from build123d import *

# Parameters (mm, degrees)
SKETCH1_R               = 7.5
BOSS_EXTRUDE1_DEPTH     = 56
SKETCH2_W               = 10
SKETCH2_H               = 16
CUT_EXTRUDE1_DEPTH      = 10
CUT_EXTRUDE4_DEPTH      = 57.995613866
CUT_EXTRUDE4_DEPTH_BACK = 57.995613866
CUT_EXTRUDE5_DEPTH      = 57.995613991
CUT_EXTRUDE5_DEPTH_BACK = 57.995613991
SKETCH4_R               = 1.5
FILLET1_R               = 0.1
SKETCH5_W               = 7.5
SKETCH5_H               = 20
SKETCH6_W               = 40
SKETCH6_H               = 40
BOSS_EXTRUDE2_DEPTH     = 5


with BuildPart() as part:
    # Sketch1 → Boss-Extrude1 (new body)
    with BuildSketch(Plane.XY):
        Circle(SKETCH1_R)
    extrude(amount=BOSS_EXTRUDE1_DEPTH)

    # Sketch2 → Cut-Extrude1 (cut)
    with BuildSketch(Plane.XY.offset(56)):
        Rectangle(SKETCH2_W, SKETCH2_H)
    extrude(amount=-CUT_EXTRUDE1_DEPTH, mode=Mode.SUBTRACT)

    # Sketch3 → Cut-Extrude4 (cut, two sides: drawn at the far end of the back side and taken through both)
    with BuildSketch(Plane(origin=(0, 0, 0), x_dir=(0, 0, -1), z_dir=(1, 0, 0)).offset(-CUT_EXTRUDE4_DEPTH_BACK)):
        with BuildLine():
            Line((-46, -114.267763227), (-46, -7.5))
            Line((-46, -7.5), (-46, -5.590169944))
            Line((-46, -5.590169944), (-52.952744721, -3.885047998))
            ThreePointArc((-52.952744721, -3.885047998), (-55.999999999, -0.000262165), (-52.952923855, 3.884664175))
            Line((-52.952923855, 3.884664175), (-46, 5.590169944))
            Line((-46, 5.590169944), (-46, 7.5))
            Line((-46, 7.5), (-46, 114.267763227))
            Line((-46, 114.267763227), (-259.535526454, 114.267763227))
            Line((-259.535526454, 114.267763227), (-259.535526454, -114.267763227))
            Line((-259.535526454, -114.267763227), (-46, -114.267763227))
        make_face()
    extrude(amount=CUT_EXTRUDE4_DEPTH + CUT_EXTRUDE4_DEPTH_BACK, mode=Mode.SUBTRACT)

    # Sketch4 → Cut-Extrude5 (cut, two sides: drawn at the far end of the back side and taken through both)
    with BuildSketch(Plane(origin=(0, 0, 0), x_dir=(0, 0, -1), z_dir=(1, 0, 0)).offset(-CUT_EXTRUDE5_DEPTH_BACK)):
        with Locations(Location((-52, -0.000169944, 0), (0, 0, 0.006491373))):
            Circle(SKETCH4_R)
    extrude(amount=CUT_EXTRUDE5_DEPTH + CUT_EXTRUDE5_DEPTH_BACK, mode=Mode.SUBTRACT)

    # Fillet1
    # the kernel refuses this fillet: 0.1 mm, written as the material it takes off along each edge
    with BuildSketch(Plane(origin=(0, 0, 46), x_dir=(0.6911452834399255, -0.7227158481580054, 0), z_dir=(0.7227158481580054, 0.6911452834399255, 0))) as fillet1_piece_1_section:
        with BuildLine():
            CenterArc((7.5 - FILLET1_R, FILLET1_R), FILLET1_R, 270, 90)
            Line((7.5 - FILLET1_R, 0), (7.5, 0))
            Line((7.5, 0), (7.5, FILLET1_R))
        make_face()
    fillet1_piece_1 = revolve(axis=Axis((0, 0, 46), (0, 0, -1)), revolution_arc=87.441672972, mode=Mode.PRIVATE)
    fillet1_piece_1 = split(fillet1_piece_1, bisect_by=Plane(origin=(5, -5.569278278, 45.983069625), z_dir=(-1, 0, 0)), keep=Keep.TOP, mode=Mode.PRIVATE)
    fillet1_piece_1 = split(fillet1_piece_1, bisect_by=Plane(origin=(-5, -5.569278278, 45.983069625), z_dir=(1, 0, 0)), keep=Keep.TOP, mode=Mode.PRIVATE)
    add(fillet1_piece_1, mode=Mode.SUBTRACT)
    with BuildSketch(Plane(origin=(0, 0, 46), x_dir=(-0.6911452834399255, 0.7227158481580054, 0), z_dir=(-0.7227158481580054, -0.6911452834399255, 0))) as fillet1_piece_2_section:
        with BuildLine():
            CenterArc((7.5 - FILLET1_R, FILLET1_R), FILLET1_R, 270, 90)
            Line((7.5 - FILLET1_R, 0), (7.5, 0))
            Line((7.5, 0), (7.5, FILLET1_R))
        make_face()
    fillet1_piece_2 = revolve(axis=Axis((0, 0, 46), (0, 0, -1)), revolution_arc=87.441672972, mode=Mode.PRIVATE)
    fillet1_piece_2 = split(fillet1_piece_2, bisect_by=Plane(origin=(5, 5.569279246, 45.98306893), z_dir=(-1, 0, 0)), keep=Keep.TOP, mode=Mode.PRIVATE)
    fillet1_piece_2 = split(fillet1_piece_2, bisect_by=Plane(origin=(-5, 5.569279246, 45.98306893), z_dir=(1, 0, 0)), keep=Keep.TOP, mode=Mode.PRIVATE)
    add(fillet1_piece_2, mode=Mode.SUBTRACT)

    # Sketch5 → Revolve1 (revolve)
    with BuildSketch(Plane(origin=(0, 0, 0), x_dir=(1, 0, 0), z_dir=(0, 1, 0)), mode=Mode.PRIVATE) as revolve1_sk:
        with Locations((-3.75, 10)):
            Rectangle(SKETCH5_W, SKETCH5_H)
    revolve(revolve1_sk.sketch.rotate(Axis((0, 0, 0), (0, 0, -1)), 31.195191598), axis=Axis((0, 0, 0), (0, 0, -1)))

    # Sketch6 → Boss-Extrude2 (add)
    with BuildSketch(Plane(origin=(0, 0, -20), x_dir=(-1, 0, 0), z_dir=(0, 0, -1))):
        Rectangle(SKETCH6_W, SKETCH6_H)
    extrude(amount=BOSS_EXTRUDE2_DEPTH)


solid = part.part
The model under review builds one solid part; all positions refer to its coordinate system, in mm. A direction names the side the tool comes from. Coordinates: 2 decimals unless noted, no trailing zeros. Write each loop counter-clockwise with the first axis right and the second up, starting at its lowest first coordinate (ties: lowest second). Pieces come first, ordered by that corner, then holes. Notation, with made-up numbers: (-27.5, 20) -> (-12.5, 20) arc R13 cw to (-12.5, 30) -> close; hole circle Ø1 at (21.5, -20.75). An arc over 180 degrees is marked (long way). Answer in a Markdown table with one row per item.
1. Wall thickness on probe 1 along Z at (x, y) = (17, -6); probe 2 along X at (y, z) = (-1, 50); probe 3 along Z at (x, y) = (4, -2.5): over which ranges is each line inside the solid? List them lowest first. Write a range as [from, to].
Answers below:
| item | result |
|---|---|
| probe 1 | z = [-25, -20] |
| probe 2 | x = [-7.43, -5], [5, 7.43] |
| probe 3 | z = [-25, 46] |
2. Clearance check with flat-ended pins moving along their axes: pin 1 Ø1 at (y, z) = (-4, -16) entering from -X; pin 2 Ø1 at (x, z) = (0.5, 24.5) entering from -Y; pin 3 Ø6 at (x, y) = (-3, 2) entering from +Z; pin 4 Ø8 at (x, y) = (-7.5, 14.5) entering from +Z. State where each tip first meets the part, or that it passes through.
Answers below:
| item | result |
|---|---|
| pin 1 | stops at x = -6.63 |
| pin 2 | stops at y = -7.5 |
| pin 3 | stops at z = 56 |
| pin 4 | stops at z = -20 |
3. We need section D-D, the plane y = 16.5. State the section outline as (x, z) points, and give its area (3 significant figures).
Answers below:
| item | result |
|---|---|
| outline | (-20, -25) -> (20, -25) -> (20, -20) -> (-20, -20) -> close |
| area | 200 mm^2 |
4. We need section B-B, the plane x = 0. State the section outline as (y, z) points.
Answers below:
| item | result |
|---|---|
| outline | (-20, -25) -> (20, -25) -> (20, -20) -> (7.5, -20) -> (7.5, 45.9) arc R0.1 ccw to (7.4, 46) -> (-7.4, 46) arc R0.1 ccw to (-7.5, 45.9) -> (-7.5, -20) -> (-20, -20) -> close |
5. For faces 1 (the flat face through (-9, 0, -20)), 2 (the flat face through (5, 0, 50)), 3 (the flat face through (-5.56, -4.56, 50.2)), list the 3-axis set-ups (+Z, -Z, +X, -X, +Y, -Y) from which the entire face can be reached by the end or side of a thin tool; tool diameter is ignored.
Answers below:
| item | result |
|---|---|
| face 1 | +Z |
| face 2 | +Z, +Y, -Y |
| face 3 | +Z, +X, -X, -Y |
6. Draft analysis for pull direction Z (two halves, no side actions). For faces 4 (the cylindrical face through (-6.269, 1.487, 52.195)), 5 (the flat face through (0, 0, -25)), 6 (the cylindrical face through (6.23, 0.45, 50.57)), 7 (the flat face through (5.54, -4.56, 50.2)), state which applies: +Z half, -Z half, draft (parallel to the pull), parting line (faces both ways), or undercut.
Answers below:
| item | result |
|---|---|
| face 4 | undercut |
| face 5 | -Z half |
| face 6 | undercut |
| face 7 | +Z half |
7. We need section C-C, the plane z = 52. State the section outline as (x, y) points, and give its area (3 significant figures).
Answers below:
| item | result |
|---|---|
| outline | (-7.35, -1.5) arc R7.5 ccw to (-6.27, -4.12) -> (-5, -4.12) -> (-5, -1.5) -> close; (-7.35, 1.5) -> (-5, 1.5) -> (-5, 4.12) -> (-6.27, 4.12) arc R7.5 ccw to start; (5, -4.12) -> (6.27, -4.12) arc R7.5 ccw to (7.35, -1.5) -> (5, -1.5) -> close; (5, 1.5) -> (7.35, 1.5) arc R7.5 ccw to (6.27, 4.12) -> (5, 4.12) -> close |
| area | 20.0 mm^2 |
8. We need section A-A, the plane y = 0. State the section outline as (x, z) points.
Answers below:
| item | result |
|---|---|
| outline | (-20, -25) -> (20, -25) -> (20, -20) -> (7.5, -20) -> (7.5, 50.5) -> (5, 50.5) -> (5, 46) -> (-5, 46) -> (-5, 50.5) -> (-7.5, 50.5) -> (-7.5, -20) -> (-20, -20) -> close; (-7.5, 53.5) -> (-5, 53.5) -> (-5, 56) -> (-7.5, 56) -> close; (5, 53.5) -> (7.5, 53.5) -> (7.5, 56) -> (5, 56) -> close |
